Part model, mm, in its own coordinate system. A direction names the side the tool comes from. Coordinates: 2 decimals unless noted, no trailing zeros. Loops run counter-clockwise (first coordinate to the right, second up) from the corner with the lowest first, then second, coordinate; pieces in that order, holes last. Notation, with made-up numbers: (9.25, 88.5) - (17.25, 88.5) arc R18 ccw to (17.25, 103.5) - close; hole circle Ø10 at (-16, 87). An arc over 180 degrees is marked (long way). Use a Markdown table: item, result. Add a question column.
1) Tool access for faces 1 (the face through (-3.99, -14.79, 22.89)), 2 (the face through (-7.5, -15, 52)), 3 (the face through (-7, -11, -22)), 4 (the face through (-2, -15, -18)): list every direction of +Z, -Z, +X, -X, +Y, -Y with a clear straight run to the whole face (end or side of a thin tool).
2) Drop flat-ended pins along their axis: P1, Ø5, axis at y = -21.5, z = -17.5, coming from the +X side; P2, Ø10, axis at x = 1.5, z = 42, coming from the +Y side; P3, Ø1.5, axis at y = -17.5, z = 12.5, coming from the +X side; P4, Ø3, axis at y = -16.5, z = 25.5, coming from the -X side. Give the stop position or say it passes through.
3) Pull direction Y, two halves, no side cores. Call faces 5 (the face through (2, -15, -18)), 6 (the face through (4.5, -16.8, -19.9)), 7 (the face through (0.54, -17.44, 58.92)): +Y half, -Y half, draft (parallel to the pull), parting line (faces both ways), or undercut.
4) Probe probe 1 along Y at (x, z) = (0, 55.5); probe 2 along X at (y, z) = (-11.5, -26); probe 3 along Z at (x, y) = (3.95, -15). List the from-to ranges inside material, lowest first. Write a range as [from, to].
5) Band-saw the part on A-A (z = -16). Give the cut face in (x, y).
6) Band-saw the part on B-B (x = 23). Give the cut face in (y, z), plus the area to 3 significant figures.
7) Band-saw the part on C-C (y = -9). Give the cut face in (x, z), plus the area to 3 significant figures.
8) Band-saw the part on D-D (z = 48). Give the cut face in (x, y).
from build123d import *

# Parameters (mm, degrees)
F0_W     = 15
F0_H     = 25
F1_DEPTH = 30
F3_D     = 5
F3_DEPTH = 12
F3_TIP   = 1.5021515476
F4_R     = 2.5
F5_DEPTH = 25
F7_DEPTH = 40


with BuildPart() as f1:
    # F0 (on Front) → F1 (new body)
    with BuildSketch(Plane.XZ):
        with BuildLine():
            Line((18.0940107676, 31.3397459622), (15.5940107676, 27.0096189432))
            ThreePointArc((15.5940107676, 27.0096189432), (30.5940107676, 27.0096189432), (38.0940107676, 40))
            ThreePointArc((38.0940107676, 40), (23.0940107676, 55), (8.0940107676, 40))
            Line((8.0940107676, 40), (13.0940107676, 40))
            ThreePointArc((13.0940107676, 40), (23.0940107676, 50), (33.0940107676, 40))
            ThreePointArc((33.0940107676, 40), (28.0940107676, 31.3397459622), (18.0940107676, 31.3397459622))
        make_face()
        with BuildLine():
            ThreePointArc((-8.0940107676, 40), (-36.0843918244, 47.5), (-15.5940107676, 27.0096189432))
            Line((-15.5940107676, 27.0096189432), (-18.0940107676, 31.3397459622))
            ThreePointArc((-18.0940107676, 31.3397459622), (-31.7542648054, 45), (-13.0940107676, 40))
            Line((-13.0940107676, 40), (-8.0940107676, 40))
        make_face()
        with BuildLine():
            ThreePointArc((-2, -14.8660687473), (-4.5705202893, -14.2867191575), (-7, -13.2664991614))
            Line((-7, -13.2664991614), (-7, -30))
            Line((-7, -30), (-2, -30))
            Line((-2, -30), (-2, -14.8660687473))
        make_face()
        with BuildLine():
            Line((7, -30), (7, -13.2664991614))
            ThreePointArc((7, -13.2664991614), (4.5705202893, -14.2867191575), (2, -14.8660687473))
            Line((2, -14.8660687473), (2, -30))
            Line((2, -30), (7, -30))
        make_face()
        with BuildLine():
            ThreePointArc((-7, -7.1414284285), (-9.9208513844, 1.2556702624), (-5, 8.6602540378))
            Line((-5, 8.6602540378), (-7.5, 12.9903810568))
            ThreePointArc((-7.5, 12.9903810568), (-14.9972810769, -0.2855876432), (-7, -13.2664991614))
            Line((-7, -13.2664991614), (-7, -7.1414284285))
        make_face()
        with BuildLine():
            ThreePointArc((5, 8.6602540378), (8.6602540378, 5), (10, 0))
            ThreePointArc((10, 0), (9.2195444573, -3.8729833462), (7, -7.1414284285))
            Line((7, -7.1414284285), (7, -13.2664991614))
            ThreePointArc((7, -13.2664991614), (12.8452325787, -7.7459666924), (15, 0))
            ThreePointArc((15, 0), (12.9903810568, 7.5), (7.5, 12.9903810568))
            Line((7.5, 12.9903810568), (5, 8.6602540378))
        make_face()
        with BuildLine():
            ThreePointArc((8.0940107676, 40), (10.1036297108, 32.5), (15.5940107676, 27.0096189432))
            Line((15.5940107676, 27.0096189432), (18.0940107676, 31.3397459622))
            ThreePointArc((18.0940107676, 31.3397459622), (14.4337567297, 35), (13.0940107676, 40))
            Line((13.0940107676, 40), (8.0940107676, 40))
        make_face()
        with BuildLine():
            Line((-18.0940107676, 31.3397459622), (-15.5940107676, 27.0096189432))
            ThreePointArc((-15.5940107676, 27.0096189432), (-10.1036297108, 32.5), (-8.0940107676, 40))
            Line((-8.0940107676, 40), (-13.0940107676, 40))
            ThreePointArc((-13.0940107676, 40), (-14.4337567297, 35), (-18.0940107676, 31.3397459622))
        make_face()
        with BuildLine():
            Line((-15.5940107676, 27.0096189432), (-7.5, 12.9903810568))
            ThreePointArc((-7.5, 12.9903810568), (-3.8822856765, 14.4888873943), (0, 15))
            Line((0, 15), (-7.5, 15))
            Line((-7.5, 15), (-7.5, 40))
            Line((-7.5, 40), (-8.0940107676, 40))
            ThreePointArc((-8.0940107676, 40), (-10.1036297108, 32.5), (-15.5940107676, 27.0096189432))
        make_face()
        with BuildLine():
            ThreePointArc((-5, 8.6602540378), (0, 10), (5, 8.6602540378))
            Line((5, 8.6602540378), (7.5, 12.9903810568))
            ThreePointArc((7.5, 12.9903810568), (3.8822856765, 14.4888873943), (0, 15))
            ThreePointArc((0, 15), (-3.8822856765, 14.4888873943), (-7.5, 12.9903810568))
            Line((-7.5, 12.9903810568), (-5, 8.6602540378))
        make_face()
        with BuildLine():
            ThreePointArc((-2, -9.7979589711), (-4.6919386858, -8.8309518948), (-7, -7.1414284285))
            Line((-7, -7.1414284285), (-7, -13.2664991614))
            ThreePointArc((-7, -13.2664991614), (-4.5705202893, -14.2867191575), (-2, -14.8660687473))
            Line((-2, -14.8660687473), (-2, -9.7979589711))
        make_face()
        with BuildLine():
            Line((7, -13.2664991614), (7, -7.1414284285))
            ThreePointArc((7, -7.1414284285), (4.6919386858, -8.8309518948), (2, -9.7979589711))
            Line((2, -9.7979589711), (2, -14.8660687473))
            ThreePointArc((2, -14.8660687473), (4.5705202893, -14.2867191575), (7, -13.2664991614))
        make_face()
        Polygon((-7.5, 15), (0, 15), (7.5, 15), (7.5, 40), (-7.5, 40), align=None)
        with Locations((0, 52.5)):
            Rectangle(F0_W, F0_H)
        with BuildLine():
            ThreePointArc((0, 15), (3.8822856765, 14.4888873943), (7.5, 12.9903810568))
            Line((7.5, 12.9903810568), (15.5940107676, 27.0096189432))
            ThreePointArc((15.5940107676, 27.0096189432), (10.1036297108, 32.5), (8.0940107676, 40))
            Line((8.0940107676, 40), (7.5, 40))
            Line((7.5, 40), (7.5, 15))
            Line((7.5, 15), (0, 15))
        make_face()
    extrude(amount=F1_DEPTH)

    # F3
    with Locations(Plane.XY.offset(65)):
        with Locations((0, -15)):
            Hole(F3_D / 2, depth=F3_DEPTH)
            with Locations((0, 0, -(F3_DEPTH + F3_TIP / 2))):  # 118° drill point
                Cone(0, F3_D / 2, F3_TIP, mode=Mode.SUBTRACT)

    # F4 (on face) → F5 (cut)
    with BuildSketch(Plane.YZ.offset(7)):
        with Locations((-15, -21.6332495807)):
            Circle(F4_R)
    extrude(amount=-F5_DEPTH, mode=Mode.SUBTRACT)

    # F6 (on face) → F7 (cut)
    with BuildSketch(Plane(origin=(0, 0, 0), x_dir=(-1, 0, 0), z_dir=(0, 1, 0))):
        Polygon((-7.5, 31), (0, 15), (8.0940107676, 31), align=None)
    extrude(amount=-F7_DEPTH, mode=Mode.SUBTRACT)


solid = f1.part
Answer block:
| question | item | result |
|---|---|---|
| 1 | face 1 | +Y, -Y |
| 1 | face 2 | +Z, +Y, -Y |
| 1 | face 3 | -Z, -X, +Y, -Y |
| 1 | face 4 | -Z, +Y, -Y |
| 2 | P1 | x = 7 |
| 2 | P2 | y = 0 |
| 2 | P3 | x = 9.32 |
| 2 | P4 | x = -30.58 |
| 3 | face 5 | draft |
| 3 | face 6 | undercut |
| 3 | face 7 | undercut |
| 4 | probe 1 | [-30, -17.5], [-12.5, 0] |
| 4 | probe 2 | [-7, -2], [2, 7] |
| 4 | probe 3 | [-30, -24.13], [-19.13, -9.19], [9.19, 23.43], [31, 65] |
| 5 | outline | (-7, -30) - (-2, -30) - (-2, 0) - (-7, 0) - close; (2, -30) - (7, -30) - (7, 0) - (2, 0) - close |
| 6 | outline | (-30, 25) - (0, 25) - (0, 30) - (-30, 30) - close; (-30, 50) - (0, 50) - (0, 55) - (-30, 55) - close |
| 6 | area | 300 mm2 |
| 7 | outline | (-15.59, 27.01) - (-7.5, 12.99) arc R15 ccw to (-7, -13.27) - (-7, -30) - (-2, -30) - (-2, -9.8) arc R10 cw (long way) to (2, -9.8) - (2, -30) - (7, -30) - (7, -13.27) arc R15 ccw to (7.5, 12.99) - (15.59, 27.01) arc R15 ccw (long way) to (8.09, 40) - (7.5, 40) - (7.5, 65) - (-7.5, 65) - (-7.5, 40) - (-8.09, 40) arc R15 ccw (long way) to start; hole circle Ø20 at (-23.09, 40); hole (-8.09, 31) - (0, 15) - (7.5, 31) - close; hole circle Ø20 at (23.09, 40) |
| 7 | area | 2,140 mm2 |
| 8 | outline | (-35.78, -30) - (-29.09, -30) - (-29.09, 0) - (-35.78, 0) - close; (-17.09, -30) - (-10.41, -30) - (-10.41, 0) - (-17.09, 0) - close; (-7.5, -30) - (7.5, -30) - (7.5, 0) - (-7.5, 0) - close; (10.41, -30) - (17.09, -30) - (17.09, 0) - (10.41, 0) - close; (29.09, -30) - (35.78, -30) - (35.78, 0) - (29.09, 0) - close |
